Part model, mm, in its own coordinate system. A direction names the side the tool comes from. Give positions to 0.01 mm unless a question says otherwise; leave off trailing zeros. Order: outer loops, then holes, each group sorted by start corner. A loop starts at its lowest first (then second) coordinate and runs counter-clockwise, first axis right, second up. Notation, with made-up numbers: (-20, 81) - (0, 81) arc R22 cw to (0, 90) - close; hole circle Ø6 at (56, -23). An arc over 180 degrees is marked (long way). Use one line per item in the form item = value. Start each with the question number.
1. Tool access for faces 1 (the face through (-17, -15, 26)), 2 (the face through (0, 1, 0)), 3 (the face through (-17.45, 25.5, 34.27)): list every direction of +Z, -Z, +X, -X, +Y, -Y with a clear straight run to the whole face (end or side of a thin tool).
2. Band-saw the part on A-A, the plane y = -42. State how many separate pieces and enclosed holes the cut face has, plus the area to 3 significant figures.
3. Drill centre lines: line 1 (Y direction, x = 0, z = 1); line 2 (X direction, y = -66.5, z = 38.5); line 3 (Z direction, x = 4, y = 19.5). Where is each one in solid material? Low to high.
4. Band-saw the part on B-B, the plane x = 0. List the corners of the cut face in (y, z).
5. Pin check, flat tips, straight feed: P1, Ø13, axis at y = -42, z = 30, coming from the -X side; P2, Ø4, axis at x = 5.5, y = -7.5, coming from the +Z side; P3, Ø18.5, axis at y = -42, z = 30, coming from the +X side. Stop position of each tip, or through.
6. Band-saw the part on D-D, the plane x = -9. List the corners of the cut face in (y, z).
from build123d import *

# Parameters (mm, degrees)
SZKIC1_W                    = 40
SZKIC1_H                    = 149
DODANIE_WYCI_GNI_CIE1_DEPTH = 60
SZKIC2_W                    = 34
SZKIC2_H                    = 57
WYTNIJ_WYCI_GNI_CIE1_DEPTH  = 162.867229543
SZKIC4_R                    = 8
WYTNIJ_WYCI_GNI_CIE2_DEPTH  = 45
SZKIC5_R                    = 4
WYTNIJ_WYCI_GNI_CIE3_DEPTH  = 96.912720741
ZAOKR_GLENIE1_R             = 1.5


with BuildPart() as part:
    # Szkic1 → Dodanie-wyciągnięcie1 (new body)
    with BuildSketch(Plane.XY):
        Rectangle(SZKIC1_W, SZKIC1_H)
    extrude(amount=DODANIE_WYCI_GNI_CIE1_DEPTH)

    # Szkic2 → Wytnij-wyciągnięcie1 (cut, through all)
    with BuildSketch(Plane(origin=(0, 74.5, 0), x_dir=(1, 0, 0), z_dir=(0, 1, 0))):
        with Locations((0, -31.5)):
            Rectangle(SZKIC2_W, SZKIC2_H)
    extrude(amount=-WYTNIJ_WYCI_GNI_CIE1_DEPTH, mode=Mode.SUBTRACT)

    # Szkic4 → Wytnij-wyciągnięcie2 (cut)
    with BuildSketch(Plane.ZY.offset(20)):
        Polygon((10, 74.5), (60, -24.5), (60, 74.5), align=None)
        with Locations((30, -42)):
            Circle(SZKIC4_R)
    extrude(amount=-WYTNIJ_WYCI_GNI_CIE2_DEPTH, mode=Mode.SUBTRACT)

    # Szkic5 → Wytnij-wyciągnięcie3 (cut, through all)
    with BuildSketch(Plane.XY.offset(3)):
        with Locations((0, 61.5)):
            Circle(SZKIC5_R)
        with Locations((0, 34.5)):
            Circle(SZKIC5_R)
        with Locations((0, 7.5)):
            Circle(SZKIC5_R)
    extrude(amount=-WYTNIJ_WYCI_GNI_CIE3_DEPTH, mode=Mode.SUBTRACT)

    # Zaokrąglenie1
    zaokr_glenie1_edges = [part.edges().sort_by_distance(p)[0] for p in [
        (0, 74.5, 3),
        (0, -74.5, 3),
        (20, 74.5, 5),
        (20, 0, 0),
        (20, -74.5, 30),
        (20, -49.5, 60),
        (20, 25, 35),
        (20, -42, 22),
        (17, -49.5, 60),
        (17, -74.5, 31.5),
        (17, 0, 3),
        (17, 74.5, 6.5),
        (17, 25, 35),
        (17, -42, 22),
        (-17, 74.5, 6.5),
        (-17, 0, 3),
        (-17, -74.5, 31.5),
        (-17, -49.5, 60),
        (-17, 25, 35),
        (-17, -42, 22),
        (-20, -49.5, 60),
        (-20, -74.5, 30),
        (-20, 0, 0),
        (-20, 74.5, 5),
        (-20, 25, 35),
        (-20, -42, 22),
    ]]
    fillet(zaokr_glenie1_edges, radius=ZAOKR_GLENIE1_R - 0.0001)  # a hair under: the kernel refuses the full size


solid = part.part
From the geometry:
q1.face_1 = +Z, +Y, -Y
q1.face_2 = -Z, +X, -X, +Y, -Y
q1.face_3 = +Z, +Y
q2.separate_pieces = 3
q2.enclosed_holes = 0
q2.area = 360 mm²
q3.line_1 = -74.5 to 3.5, 11.5 to 30.5, 38.5 to 57.5, 65.5 to 74.5
q3.line_2 = -20 to -17, 17 to 20
q3.line_3 = 0 to 3
q4.outline = (-74.5, 0) - (3.5, 0) - (3.5, 3) - (-73, 3) arc R1.5 ccw to (-74.5, 1.5) - close; (11.5, 0) - (30.5, 0) - (30.5, 3) - (11.5, 3) - close; (38.5, 0) - (57.5, 0) - (57.5, 3) - (38.5, 3) - close; (65.5, 0) - (74.5, 0) - (74.5, 1.5) arc R1.5 ccw to (73, 3) - (65.5, 3) - close
q5.P1 = through
q5.P2 = 3
q5.P3 = 19.98
q6.outline = (-74.5, 0) - (74.5, 0) - (74.5, 1.5) arc R1.5 ccw to (73, 3) - (-73, 3) arc R1.5 ccw to (-74.5, 1.5) - close
